```python
from build123d import *


with BuildPart() as f1:
    # F0 (on Front) → F1 (revolve)
    with BuildSketch(Plane.XZ):
        with BuildLine():
            Line((0, 3.175), (0, 0))
            Line((0, 0), (51.181, 0))
            ThreePointArc((51.181, 0), (51.046133, 2.024703), (50.643913, 4.01363))
            ThreePointArc((50.643913, 4.01363), (50.280446, 4.55386), (49.663659, 4.7625))
            Line((49.663659, 4.7625), (48.26, 4.7625))
            ThreePointArc((48.26, 4.7625), (47.54158, 4.46492), (47.244, 3.7465))
            Line((47.244, 3.7465), (47.244, 3.175))
            Line((47.244, 3.175), (0, 3.175))
        make_face()
    revolve(axis=Axis((25.5905, 0, 0), (1, 0, 0)))

    # F2: F1 across plane


with BuildPart() as f1_1:
    add(f1.part)
    add(f1.part.mirror(Plane.YZ))


solid = f1_1.part
```
Here's how the part is built. I have some questions about the finished solid (model axes, mm). Round coordinates to 2 decimals unless told otherwise and drop trailing zeros. Write each loop counter-clockwise with the first axis right and the second up, starting at its lowest first coordinate (ties: lowest second). Pieces come first, ordered by that corner, then holes.
Q1. Please list where these lines run through material, in increasing order: probe 1 along Y at (x, z) = (-28.5, 0) (3 decimals); probe 2 along X at (y, z) = (-1.25, 3.5).
Q2. Will these pins go through, and if not, where does the flat tip stop? P1, Ø2, axis at x = -14.5, z = -0.5, coming from the -Y side (3 decimals); P2, Ø2, axis at y = -1.5, z = 1.5, coming from the -X side; P3, Ø5, axis at x = -13.5, y = 0, coming from the +Z side (3 decimals).
Q3. If we mould it in two halves opening along X, with no side actions, what happens to faces 1 (the cylindrical face through (-48.95, 2.9, -3.78)), 2 (the cylindrical face through (0.66, 3.1, -0.69))? For each: +X half, -X half, draft (parallel to the pull), parting line (faces both ways), or undercut.
Q4. If we section it at A-A on x = 19: Write out the boundary of the cut face in (y, z) (3 decimals), plus the area to 3 significant figures.
Answer below:
1. probe 1: y = -3.175 to 3.175
1. probe 2: x = -50.72 to -47.24, 47.24 to 50.72
2. P1: stops at y = -3.175
2. P2: stops at x = -51.14
2. P3: stops at z = 3.175
3. face 1: draft
3. face 2: undercut
4. outline: circle Ø6.35 at (0, 0)
4. area: 31.7 mm2
